Can you work these out from the model? Positions are in its coordinate system, mm. A direction names the side the tool comes from. Coordinates: 2 decimals unless noted, no trailing zeros. Write each loop counter-clockwise with the first axis right and the second up, starting at its lowest first coordinate (ties: lowest second). Pieces come first, ordered by that corner, then holes. Notation, with made-up numbers: (29, 26.25) - (63, 26.25) arc R13 cw to (63, 51.25) - close; hole circle Ø9 at (12, -5). An arc over 180 degrees is marked (long way). Use one line per item in the form item = value. Start each with the question number.
(1) On a 3-axis mill with a long thin cutter (end or side, diameter ignored), from which of +Z, -Z, +X, -X, +Y, -Y can I reach the whole of each face in a straight line? I mean faces 1 (the face through (157.8, 66.6, 6.5)), 2 (the face through (157.275, 70.613, 3.965)). Say none if no direction works.
(2) If we section it at A-A on x = 163.5: Please give me the cut outline in (y, z).
(3) If we section it at C-C on y = 65.5: Please give me the cut outline in (x, z).
(4) Thinking about a two-plate mould opening in X: for faces 3 (the face through (171.583, 68, 1)), 4 (the face through (165.242, 70.993, 0.74)), 5 (the face through (157.275, 66.613, 3.965)), 6 (the face through (164, 62.591, 1)), which applies, pulls with the +X half, pulls with the -X half, needs draft (parallel to the pull), parting line crosses it, or undercut?
(5) If we section it at B-B on y = 69.5: Please give me the cut outline in (x, z).
(6) For pin 1 Ø3.5 at (x, y) = (163.81, 70.54) entering from +Z; pin 2 Ø1.5 at (x, z) = (159.5, 4.5) entering from +Y, each with a flat end and sliding along its axis, tell me the tip position at first contact or that it passes through.
(7) If we section it at D-D on x = 160.25: Please give me the cut outline in (y, z), then the cut area to 3 significant figures.
(8) If I drill on probe 1 along Y at (x, z) = (157.75, 1.75); probe 2 along Z at (x, y) = (157.5, 63); probe 3 along Y at (x, z) = (158, 3.25), over which ranges is the centre line in solid material (lowest first)? Write a range as from..to.
```python
from build123d import *

# Parameters (mm, degrees)
SKETCH1_W           = 15
SKETCH1_H           = 10
SKETCH1_R           = 1.5
BOSS_EXTRUDE1_DEPTH = 1.5
SKETCH2_R           = 0.5
BOSS_EXTRUDE2_DEPTH = 5


with BuildPart() as part:
    # Sketch1 → Boss-Extrude1 (new body)
    with BuildSketch(Plane.XY):
        with Locations((164.083059714, 67.591147655)):
            Rectangle(SKETCH1_W, SKETCH1_H)
        with Locations((163.811741983, 70.542925262)):
            Circle(SKETCH1_R, mode=Mode.SUBTRACT)
    extrude(amount=BOSS_EXTRUDE1_DEPTH)

    # Sketch2 → Boss-Extrude2 (add)
    with BuildSketch(Plane.XY.offset(1.5)):
        with Locations((157.774202419, 68.591147655)):
            Circle(SKETCH2_R)
        with Locations((157.774202419, 70.591147655)):
            Circle(SKETCH2_R)
        with Locations((157.774202419, 64.591147655)):
            Circle(SKETCH2_R)
        with Locations((157.774202419, 66.591147655)):
            Circle(SKETCH2_R)
    extrude(amount=BOSS_EXTRUDE2_DEPTH)


solid = part.part
```
Reported:
q1.face_1 = +Z, +X, -X, +Y, -Y
q1.face_2 = +Z
q2.outline = (62.59, 0) - (69.08, 0) - (69.08, 1.5) - (62.59, 1.5) - close; (72.01, 0) - (72.59, 0) - (72.59, 1.5) - (72.01, 1.5) - close
q3.outline = (156.58, 0) - (171.58, 0) - (171.58, 1.5) - (156.58, 1.5) - close
q4.face_3 = pulls with the +X half
q4.face_4 = undercut
q4.face_5 = parting line crosses it
q4.face_6 = needs draft
q5.outline = (156.58, 0) - (162.73, 0) - (162.73, 1.5) - (156.58, 1.5) - close; (164.89, 0) - (171.58, 0) - (171.58, 1.5) - (164.89, 1.5) - close
q6.pin_1 = 1.5
q6.pin_2 = through
q7.outline = (62.59, 0) - (72.59, 0) - (72.59, 1.5) - (62.59, 1.5) - close
q7.area = 15.0 mm2
q8.probe_1 = 64.09..65.09, 66.09..67.09, 68.09..69.09, 70.09..71.09
q8.probe_2 = 0..1.5
q8.probe_3 = 64.15..65.04, 66.15..67.04, 68.15..69.04, 70.15..71.04
